Work out the finished part from the listing and answer in its coordinate system (mm). Face numbers are marked on the shaded views. A direction names the side the tool comes from. Give positions to 0.01 mm unless a question says otherwise; leave off trailing zeros. Loops run counter-clockwise (first coordinate to the right, second up) from the corner with the lowest first, then second, coordinate; pieces in that order, holes last. Notation, with made-up numbers: (-6, 44) - (41, 44) arc R27 cw to (41, 71) - close; hole circle Ø1 at (41, 37.25). An arc over 180 degrees is marked (long way). Use one line per item in the form item = value. Start each with the question number.
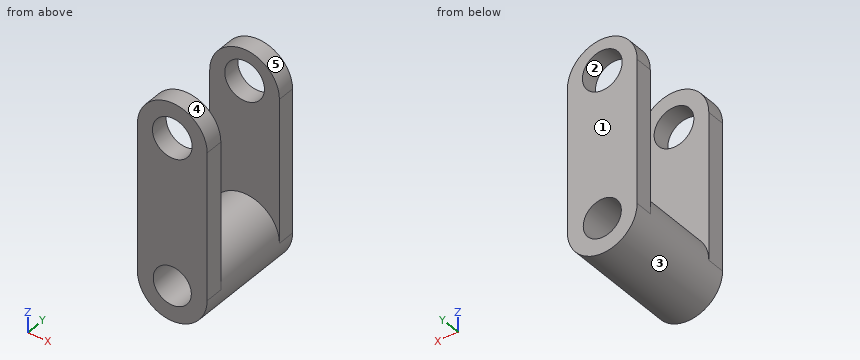
from build123d import *

# Parameters (mm, degrees)
F0_R     = 32.56316
F1_DEPTH = 108.966
F3_DEPTH = 16.764
F5_DEPTH = 17.526
F6_R     = 18.566269
F7_DEPTH = 188.214
F6_R_2   = 17.808278
F8_DEPTH = 219.202


with BuildPart() as f1:
    # F0 (on Front) → F1 (new body)
    with BuildSketch(Plane.XZ):
        Circle(F0_R)
    extrude(amount=F1_DEPTH)

    # F2 (on face) → F3 (join)
    with BuildSketch(Plane(origin=(0, 0, 0), x_dir=(-1, 0, 0), z_dir=(0, 1, 0))):
        with BuildLine():
            ThreePointArc((-32.56316, 0), (0, 32.56316), (32.56316, 0))
            Line((32.56316, 0), (32.56316, 133.426726))
            ThreePointArc((32.56316, 133.426726), (0, 165.989885), (-32.56316, 133.426726))
            Line((-32.56316, 133.426726), (-32.56316, 0))
        make_face()
    extrude(amount=-F3_DEPTH)

    # F4 (on face) → F5 (join)
    with BuildSketch(Plane.XZ.offset(108.966)):
        with BuildLine():
            Line((-32.56316, 136.865824), (-32.56316, 0))
            ThreePointArc((-32.56316, 0), (0, 32.56316), (32.56316, 0))
            Line((32.56316, 0), (32.56316, 136.865824))
            ThreePointArc((32.56316, 136.865824), (0, 169.428984), (-32.56316, 136.865824))
        make_face()
    extrude(amount=-F5_DEPTH)

    # F6 (on face) → F7 (cut)
    with BuildSketch(Plane.XZ.offset(108.966)):
        with Locations((0, 136.865824)):
            Circle(F6_R)
    extrude(amount=-F7_DEPTH, mode=Mode.SUBTRACT)

    # F6 (on face) → F8 (cut)
    with BuildSketch(Plane.XZ.offset(108.966)):
        Circle(F6_R_2)
    extrude(amount=-F8_DEPTH, mode=Mode.SUBTRACT)


solid = f1.part
1) Find the intervals of material crossed by probe 1 along Z at (x, y) = (0, -6); probe 2 along Z at (x, y) = (0, -103); probe 3 along Y at (x, z) = (-16, 58.5), in increasing order.
2) A cutting plane is placed at C-C (x = -12). Give the vertices of the cut face in (y, z), plus the area to 3 significant figures.
3) A cutting plane is placed at D-D (x = -23.5). Give the vertices of the cut face in (y, z).
4) Flat-ended cylindrical pins translate along their axes: pin 1 Ø6 at (x, y) = (17.5, -95) entering from +Z; pin 2 Ø12 at (x, y) = (-17.5, -37) entering from -Z; pin 3 Ø4 at (x, y) = (-23.5, -45.5) entering from +Z. Find the tip coordinate at first contact, or state that the pin passes through.
5) A tool of negligible diameter and unlimited length cuts with its end or side. For the marked faces 4 and 5, from which of +Z, -Z, +X, -X, +Y, -Y can it reach the whole face along a straight path? Write none if from no direction.
6) A cutting plane is placed at B-B (y = -33). Give the vertices of the cut face in (x, z), plus the area to 3 significant figures.
7) Determine the mould class of the marked faces 1, 2 and 3 for opening direction X: released by +X, released by -X, zero draft, split by the parting line, or undercut.
8) A cutting plane is placed at A-A (x = 0). Give the vertices of the cut face in (y, z), plus the area to 3 significant figures.
Answer sheet:
q1.probe_1 = -32.56 to -17.81, 17.81 to 118.3, 155.43 to 165.99
q1.probe_2 = -32.56 to -17.81, 17.81 to 118.3, 155.43 to 169.43
q1.probe_3 = -108.97 to -91.44, -16.76 to 0
q2.outline = (-108.97, -30.27) - (0, -30.27) - (0, -13.16) - (-108.97, -13.16) - close; (-108.97, 13.16) - (0, 13.16) - (0, 122.7) - (-16.76, 122.7) - (-16.76, 30.27) - (-91.44, 30.27) - (-91.44, 122.7) - (-108.97, 122.7) - close; (-108.97, 151.03) - (-91.44, 151.03) - (-91.44, 167.14) - (-108.97, 167.14) - close; (-16.76, 151.03) - (0, 151.03) - (0, 163.7) - (-16.76, 163.7) - close
q2.area = 7,390 mm²
q3.outline = (-108.97, -22.54) - (0, -22.54) - (0, 155.97) - (-16.76, 155.97) - (-16.76, 22.54) - (-91.44, 22.54) - (-91.44, 159.41) - (-108.97, 159.41) - close
q4.pin_1 = 166.02
q4.pin_2 = -30.46
q4.pin_3 = 24.46
q5.face_4 = +Z, +Y, -Y
q5.face_5 = +Z, +Y
q6.outline = circle Ø65.13 at (0, 0); hole circle Ø35.62 at (0, 0)
q6.area = 2,330 mm²
q7.face_1 = zero draft
q7.face_2 = undercut
q7.face_3 = split by the parting line
q8.outline = (-108.97, -32.56) - (0, -32.56) - (0, -17.81) - (-108.97, -17.81) - close; (-108.97, 17.81) - (0, 17.81) - (0, 118.3) - (-16.76, 118.3) - (-16.76, 32.56) - (-91.44, 32.56) - (-91.44, 118.3) - (-108.97, 118.3) - close; (-108.97, 155.43) - (-91.44, 155.43) - (-91.44, 169.43) - (-108.97, 169.43) - close; (-16.76, 155.43) - (0, 155.43) - (0, 165.99) - (-16.76, 165.99) - close
q8.area = 6,580 mm²
